Part model, mm, in its own coordinate system. Give positions to 0.01 mm unless a question says otherwise; leave off trailing zeros. Order: outer loops, then holes, each group sorted by start corner. A loop starts at its lowest first (then second) coordinate and runs counter-clockwise, first axis right, second up.
1. Slice it at B-B on y = -6. List the corners of the cut face in (x, z), and give its area (3 significant figures).
2. Probe line 1 (Z direction, x = -2.5, y = -6); line 2 (Y direction, x = -1.75, z = -5.5); line 3 (Y direction, x = -4, z = -4.75). List the from-to ranges inside material, lowest first.
3. Slice it at D-D on z = -6.5. List the corners of the cut face in (x, y), and give its area (3 significant figures).
4. Drop a flat-ended pin along its axis: pin 1 Ø3 at (y, z) = (-6, -5.85) entering from +X. Give the stop position or say it passes through.
5. Mould opens along Y. For faces 1 (the cylindrical face through (-3, 0, -6)), 2 (the flat face through (-4, 0, -0.85)), 3 (the flat face through (-4, 11, -6)) say: +Y half, -Y half, draft (parallel to the pull), parting line (faces both ways), or undercut.
6. Slice it at A-A on x = -2.25. List the corners of the cut face in (y, z), and give its area (3 significant figures).
7. Slice it at C-C on x = -3.25. List the corners of the cut face in (y, z), and give its area (3 significant figures).
Solid Edge part; units mm, degrees
sketch "Sketch1" plane through (0, 0, 0) normal (1, 0, 0) x (0, 1, 0)
  circle A0 centre (-6, -5.85) radius 1.7
  line L0 (11, -10.85) -> (-11, -10.85)
  line L1 (-11, -10.85) -> (-11, -0.85)
  line L2 (-11, -0.85) -> (11, -0.85)
  line L3 (11, -0.85) -> (11, -10.85)
  circle A1 centre (6, -5.85) radius 1.7
  dimension "D1" = 11
  dimension "D2" = 11
extrude "Protrusion1" add sketch "Sketch1" against normal blind 8
sketch "Sketch2" plane through (-5, 0, -10.85) normal (0, 0, -1) x (0, -1, 0)
  circle A0 centre (0, -5) radius 3
extrude "Cutout1" cut sketch "Sketch2" against normal through all
properties material "ABS Plastic, high impact"
Data:
1. outline: (-8, -10.85) - (0, -10.85) - (0, -7.55) - (-8, -7.55) - close; (-8, -4.15) - (0, -4.15) - (0, -0.85) - (-8, -0.85) - close
1. area: 52.8 mm2
2. line 1: z = -10.85 to -7.55, -4.15 to -0.85
2. line 2: y = -11 to -7.66, -4.34 to -2.44, 2.44 to 4.34, 7.66 to 11
2. line 3: y = -11 to -7.3, -4.7 to 4.7, 7.3 to 11
3. outline: (-8, -11) - (0, -11) - (0, -7.57) - (-8, -7.57) - close; (-8, -4.43) - (0, -4.43) - (0, -3) arc R3 cw to (0, 3) - (0, 4.43) - (-8, 4.43) - close; (-8, 7.57) - (0, 7.57) - (0, 11) - (-8, 11) - close
3. area: 112 mm2
4. pin 1: passes through
5. face 1: undercut
5. face 2: draft
5. face 3: +Y half
6. outline: (-11, -10.85) - (-1.98, -10.85) - (-1.98, -0.85) - (-11, -0.85) - close; (1.98, -10.85) - (11, -10.85) - (11, -0.85) - (1.98, -0.85) - close; hole circle Ø3.4 at (-6, -5.85); hole circle Ø3.4 at (6, -5.85)
6. area: 162 mm2
7. outline: (-11, -10.85) - (11, -10.85) - (11, -0.85) - (-11, -0.85) - close; hole circle Ø3.4 at (-6, -5.85); hole circle Ø3.4 at (6, -5.85)
7. area: 202 mm2
